```python
from build123d import *

# Parameters (mm, degrees)
SKETCH1_R           = 41.275
BOSS_EXTRUDE1_DEPTH = 165.1
SKETCH2_R           = 14.2875
CUT_EXTRUDE1_DEPTH  = 3.175
SKETCH3_R           = 6.6675
CUT_EXTRUDE2_DEPTH  = 12.7
SKETCH4_R           = 4.1275
CUT_EXTRUDE3_DEPTH  = 9.525
SKETCH5_R           = 1.9685
CUT_EXTRUDE4_DEPTH  = 19.05
CUT_EXTRUDE5_START  = -3.175
SKETCH6_R           = 14.2875
CUT_EXTRUDE5_DEPTH  = 3.175


with BuildPart() as part:
    # Sketch1 → Boss-Extrude1 (new body)
    with BuildSketch(Plane.XY):
        Circle(SKETCH1_R)
    extrude(amount=BOSS_EXTRUDE1_DEPTH)

    # Sketch2 → Cut-Extrude1 (cut)
    with BuildSketch(Plane.XY.offset(165.1)):
        Circle(SKETCH2_R)
    extrude(amount=-CUT_EXTRUDE1_DEPTH, mode=Mode.SUBTRACT)

    # Sketch3 → Cut-Extrude2 (cut)
    with BuildSketch(Plane.XY.offset(161.925)):
        Circle(SKETCH3_R)
    extrude(amount=-CUT_EXTRUDE2_DEPTH, mode=Mode.SUBTRACT)

    # Sketch4 → Cut-Extrude3 (cut)
    with BuildSketch(Plane.XY.offset(165.1)):
        with Locations((0, 31.75)):
            Circle(SKETCH4_R)
        with Locations((0, -31.75)):
            Circle(SKETCH4_R)
    extrude(amount=-CUT_EXTRUDE3_DEPTH, mode=Mode.SUBTRACT)

    # Sketch5 → Cut-Extrude4 (cut)
    with BuildSketch(Plane.XY.offset(165.1)):
        with Locations((-22.225, 22.225)):
            Circle(SKETCH5_R)
        with Locations((-22.225, -22.225)):
            Circle(SKETCH5_R)
        with Locations((22.225, -22.225)):
            Circle(SKETCH5_R)
        with Locations((22.225, 22.225)):
            Circle(SKETCH5_R)
    extrude(amount=-CUT_EXTRUDE4_DEPTH, mode=Mode.SUBTRACT)

    # Sketch6 → Cut-Extrude5 (cut)
    with BuildSketch(Plane(origin=(0, 0, 0), x_dir=(-1, 0, 0), z_dir=(0, 0, -1)).offset(CUT_EXTRUDE5_START)):
        with Locations(Location((0, 0, 0), (0, 0, 180))):
            Circle(SKETCH6_R)
    extrude(amount=CUT_EXTRUDE5_DEPTH, mode=Mode.SUBTRACT)


solid = part.part
```
Geometry: final body of the model. Coordinates: model frame, mm. A direction names the side the tool comes from. Give positions to 0.01 mm unless a question says otherwise; leave off trailing zeros. Loops run counter-clockwise (first coordinate to the right, second up) from the corner with the lowest first, then second, coordinate; pieces in that order, holes last. Notation, with made-up numbers: (37.25, 74.5) - (66.25, 74.5) arc R20 ccw to (66.25, 88.5) - close; hole circle Ø3 at (19.5, 84). An arc over 180 degrees is marked (long way). Answer as CSV lines item,"result". Start each with the question number.
(1) Section query C-C (z = 67). Output: boundary loops of the cut face in (x, y) (3 decimals), and give its area (3 significant figures).
(2) Section query B-B (x = 0). Output: boundary loops of the cut face in (y, z) (1 decimal), and give its area (3 significant figures).
(3) Mould query, pull axis Y, two halves, no side actions, for faces 4 (the face through (-8.948, -40.293, 81.394)), 5 (the face through (-1, -18, 165.1)), 6 (the face through (22, 22, 146.05)). Classes: +Y half, -Y half, draft (parallel to the pull), parting line (faces both ways), or undercut.
(4) Section query D-D (x = 11.5). Output: boundary loops of the cut face in (y, z) (3 decimals).
(5) Section query A-A (y = 0). Output: boundary loops of the cut face in (x, z) (1 decimal), and give its area (3 significant figures).
(6) Ray query, line 1 along Y through (x, z) = (0, 162.75) (1 decimal); line 2 along X through (y, z) = (23, 148.5); line 3 along X through (y, z) = (22.5, 155.5). Return the intervals inside material, ascending. Write a range as [from, to].
(7) Reachability of faces 1 (the face through (20.66, -23.42, 155.71)), 2 (the face through (0, 0, 3.175)), 3 (the face through (-1, -18, 0)) from +Z, -Z, +X, -X, +Y, -Y: full face, straight path, thin tool, end or side. Return the list, or none.
(8) Pin query (flat end, axial travel): P1, Ø4, axis at x = 9.5, z = 60.5, coming from the -Y side; P2, Ø8, axis at y = -20.5, z = 80, coming from the -X side; P3, Ø1.2, axis at x = -22, y = 22.5, coming from the +Z side. Return the tip coordinate at first contact, or that it passes through.
Worked answers:
1,outline,"circle Ø82.55 at (0, 0)"
1,area,"5,350 mm^2"
2,outline,"(-41.3, 0) - (-14.3, 0) - (-14.3, 3.2) - (14.3, 3.2) - (14.3, 0) - (41.3, 0) - (41.3, 165.1) - (35.9, 165.1) - (35.9, 155.6) - (27.6, 155.6) - (27.6, 165.1) - (14.3, 165.1) - (14.3, 161.9) - (6.7, 161.9) - (6.7, 149.2) - (-6.7, 149.2) - (-6.7, 161.9) - (-14.3, 161.9) - (-14.3, 165.1) - (-27.6, 165.1) - (-27.6, 155.6) - (-35.9, 155.6) - (-35.9, 165.1) - (-41.3, 165.1) - close"
2,area,"13,100 mm^2"
3,face 4,"parting line"
3,face 5,"draft"
3,face 6,"undercut"
4,outline,"(-39.641, 0) - (-8.478, 0) - (-8.478, 3.175) - (8.478, 3.175) - (8.478, 0) - (39.641, 0) - (39.641, 165.1) - (8.478, 165.1) - (8.478, 161.925) - (-8.478, 161.925) - (-8.478, 165.1) - (-39.641, 165.1) - close"
5,outline,"(-41.3, 0) - (-14.3, 0) - (-14.3, 3.2) - (14.3, 3.2) - (14.3, 0) - (41.3, 0) - (41.3, 165.1) - (14.3, 165.1) - (14.3, 161.9) - (6.7, 161.9) - (6.7, 149.2) - (-6.7, 149.2) - (-6.7, 161.9) - (-14.3, 161.9) - (-14.3, 165.1) - (-41.3, 165.1) - close"
5,area,"13,300 mm^2"
6,line 1,"y = [-41.3, -35.9], [-27.6, -14.3], [14.3, 27.6], [35.9, 41.3]"
6,line 2,"x = [-34.27, -24.03], [-20.42, 20.42], [24.03, 34.27]"
6,line 3,"x = [-34.6, -24.17], [-20.28, 20.28], [24.17, 34.6]"
7,face 1,"+Z"
7,face 2,"-Z"
7,face 3,"-Z, +X, -X, +Y, -Y"
8,P1,"stops at y = -40.59"
8,P2,"stops at x = -37.83"
8,P3,"stops at z = 146.05"
